from build123d import *

# Parameters (mm, degrees)
SKETCH4_W           = 25
SKETCH4_H           = 25
BOSS_EXTRUDE1_DEPTH = 35
CUT_EXTRUDE12_DEPTH = 50
SKETCH23_W          = 25
SKETCH23_H          = 22.5
CUT_EXTRUDE13_DEPTH = 7
SKETCH24_W          = 30.861916298
SKETCH24_H          = 6.481730837
BOSS_EXTRUDE6_DEPTH = 2
SKETCH25_R          = 1.5
CUT_EXTRUDE14_DEPTH = 3.5
SKETCH26_R          = 1.5
CUT_EXTRUDE15_DEPTH = 3.5
BOSS_EXTRUDE8_DEPTH = 6
SKETCH28_R          = 1.5
CUT_EXTRUDE16_DEPTH = 10
SKETCH29_R          = 1.5
CUT_EXTRUDE17_DEPTH = 10
SKETCH30_R          = 10.5
CUT_EXTRUDE18_DEPTH = 2


with BuildPart() as part:
    # Sketch4 → Boss-Extrude1 (new body)
    with BuildSketch(Plane(origin=(0, 0, 0), x_dir=(1, 0, 0), z_dir=(0, 1, 0))):
        with BuildLine():
            Line((-14.859531773, 13.748687459), (16.140468227, 13.748687459))
            ThreePointArc((16.140468227, 13.748687459), (18.261788571, 12.870007803), (19.140468227, 10.748687459))
            Line((19.140468227, 10.748687459), (19.140468227, -20.251312541))
            ThreePointArc((19.140468227, -20.251312541), (18.261788571, -22.372632884), (16.140468227, -23.251312541))
            Line((16.140468227, -23.251312541), (-14.859531773, -23.251312541))
            ThreePointArc((-14.859531773, -23.251312541), (-16.980852116, -22.372632884), (-17.859531773, -20.251312541))
            Line((-17.859531773, -20.251312541), (-17.859531773, 10.748687459))
            ThreePointArc((-17.859531773, 10.748687459), (-16.980852116, 12.870007803), (-14.859531773, 13.748687459))
        make_face()
        with Locations((0.640468227, -4.751312541)):
            Rectangle(SKETCH4_W, SKETCH4_H, mode=Mode.SUBTRACT)
    extrude(amount=BOSS_EXTRUDE1_DEPTH)

    # Sketch22 → Cut-Extrude12 (cut)
    with BuildSketch(Plane.ZY.offset(17.859531773)):
        Polygon((-13.748687459, 35), (-13.748687459, 0), (13.251312541, 0), (13.251312541, 12), (-1.748687459, 12), (-1.748687459, 6), (-7.748687459, 6), (-7.748687459, 35), align=None)
    extrude(amount=-CUT_EXTRUDE12_DEPTH, mode=Mode.SUBTRACT)

    # Sketch23 → Cut-Extrude13 (cut)
    with BuildSketch(Plane.XY.offset(23.251312541)):
        with Locations((0.640468227, 18.25)):
            Rectangle(SKETCH23_W, SKETCH23_H)
    extrude(amount=-CUT_EXTRUDE13_DEPTH, mode=Mode.SUBTRACT)

    # Sketch24 → Boss-Extrude6 (add)
    with BuildSketch(Plane.XZ):
        with Locations((1.291847829, 16.49217796)):
            Rectangle(SKETCH24_W, SKETCH24_H)
    extrude(amount=-BOSS_EXTRUDE6_DEPTH)

    # Sketch25 → Cut-Extrude14 (cut)
    with BuildSketch(Plane(origin=(0, 0, -7.748687459), x_dir=(-1, 0, 0), z_dir=(0, 0, -1))):
        with Locations((-16.140468227, 21.5)):
            Circle(SKETCH25_R)
        with Locations((-16.140468227, 17)):
            Circle(SKETCH25_R)
        with Locations((-16.140468227, 12.5)):
            Circle(SKETCH25_R)
        with Locations((14.859531773, 12.5)):
            Circle(SKETCH25_R)
        with Locations((14.859531773, 21.5)):
            Circle(SKETCH25_R)
        with Locations((14.859531773, 17)):
            Circle(SKETCH25_R)
        with Locations((14.859531773, 30.5)):
            Circle(SKETCH25_R)
        with Locations((-16.140468227, 30.5)):
            Circle(SKETCH25_R)
        with Locations((-16.140468227, 26)):
            Circle(SKETCH25_R)
        with Locations((14.859531773, 26)):
            Circle(SKETCH25_R)
    extrude(amount=-CUT_EXTRUDE14_DEPTH, mode=Mode.SUBTRACT)

    # Sketch26 → Cut-Extrude15 (cut)
    with BuildSketch(Plane.XZ.offset(-6)):
        with Locations(Location((-14.859531773, -4.748687459, 0), (0, 0, 270))):
            Circle(SKETCH26_R)
        with Locations(Location((16.140468227, -4.748687459, 0), (0, 0, 270))):
            Circle(SKETCH26_R)
    extrude(amount=-CUT_EXTRUDE15_DEPTH, mode=Mode.SUBTRACT)

    # Sketch27 → Boss-Extrude8 (add)
    with BuildSketch(Plane(origin=(0, 35, 0), x_dir=(1, 0, 0), z_dir=(0, 1, 0))):
        with BuildLine():
            Line((-14.859531773, -23.251312541), (16.140468227, -23.251312541))
            ThreePointArc((16.140468227, -23.251312541), (18.261788571, -22.372632884), (19.140468227, -20.251312541))
            Line((19.140468227, -20.251312541), (19.140468227, 10.748687459))
            ThreePointArc((19.140468227, 10.748687459), (18.261788571, 12.870007803), (16.140468227, 13.748687459))
            Line((16.140468227, 13.748687459), (-14.859531773, 13.748687459))
            ThreePointArc((-14.859531773, 13.748687459), (-16.980852116, 12.870007803), (-17.859531773, 10.748687459))
            Line((-17.859531773, 10.748687459), (-17.859531773, -20.251312541))
            ThreePointArc((-17.859531773, -20.251312541), (-16.980852116, -22.372632884), (-14.859531773, -23.251312541))
        make_face()
    extrude(amount=BOSS_EXTRUDE8_DEPTH)

    # Sketch28 → Cut-Extrude16 (cut)
    with BuildSketch(Plane.XY.offset(23.251312541)):
        with Locations((-5.609531773, 32)):
            Circle(SKETCH28_R)
        with Locations((6.890468227, 32)):
            Circle(SKETCH28_R)
        with Locations((-5.609531773, 4.5)):
            Circle(SKETCH28_R)
        with Locations((6.890468227, 4.5)):
            Circle(SKETCH28_R)
    extrude(amount=-CUT_EXTRUDE16_DEPTH, mode=Mode.SUBTRACT)

    # Sketch29 → Cut-Extrude17 (cut)
    with BuildSketch(Plane(origin=(0, 41, 0), x_dir=(1, 0, 0), z_dir=(0, 1, 0))):
        with Locations(Location((0.640468227, 2.248687459, 0), (0, 0, 270))):
            Circle(SKETCH29_R)
        with Locations(Location((7.640468227, -4.751312541, 0), (0, 0, 270))):
            Circle(SKETCH29_R)
        with Locations(Location((0.640468227, -11.751312541, 0), (0, 0, 270))):
            Circle(SKETCH29_R)
        with Locations(Location((-6.359531773, -4.751312541, 0), (0, 0, 270))):
            Circle(SKETCH29_R)
        with Locations(Location((0.640468227, -4.751312541, 0), (0, 0, 270))):
            Circle(SKETCH29_R)
    extrude(amount=-CUT_EXTRUDE17_DEPTH, mode=Mode.SUBTRACT)

    # Sketch30 → Cut-Extrude18 (cut)
    with BuildSketch(Plane(origin=(0, 41, 0), x_dir=(1, 0, 0), z_dir=(0, 1, 0))):
        with Locations(Location((0.640468227, -4.751312541, 0), (0, 0, 270))):
            Circle(SKETCH30_R)
    extrude(amount=-CUT_EXTRUDE18_DEPTH, mode=Mode.SUBTRACT)


solid = part.part
Build history of the part. All positions in model axes, mm. A direction names the side the tool comes from. Round coordinates to 2 decimals unless told otherwise and drop trailing zeros. Loops run counter-clockwise (first coordinate to the right, second up) from the corner with the lowest first, then second, coordinate; pieces in that order, holes last. Notation, with made-up numbers: (66, 32.25) -> (81, 32.25) arc R9 ccw to (81, 40.25) -> close; hole circle Ø6 at (-4.75, 0). An arc over 180 degrees is marked (long way). One line per item, written item: value. Start each with the question number.
Q1. Two-plate mould, pull along Z, no slides. Class faces 4 (the face through (-15, 12, 6)), 5 (the face through (6.176, 37.028, 4.426)), 6 (the face through (16, 17, -4.249)), 7 (the face through (7.58, 30.67, 20.29)): released by +Z, released by -Z, zero draft, split by the parting line, or undercut.
Q2. Cut at D-D on z = 8.5. List the corners of the cut face in (x, y).
Q3. Cut at C-C on x = 7. List the corners of the cut face in (y, z), plus the area to 3 significant figures.
Q4. 3-axis set-ups, long thin cutter, end or side, ignore diameter. For faces 1 (the face through (18.28, 37.96, -12.85)), 2 (the face through (16, 9, -1.749)), 3 (the face through (0, 2, 15)): which of +Z, -Z, +X, -X, +Y, -Y reach the whole face in a straight line?
Q5. Drop flat-ended pins along their axis: pin 1 Ø3.5 at (x, y) = (16, 30.5) entering from -Z; pin 2 Ø3 at (x, z) = (17, 8) entering from -Y; pin 3 Ø1.5 at (x, y) = (-14.5, 25.5) entering from -Z; pin 4 Ø5 at (x, y) = (6.89, 4.5) entering from +Z. Give the stop position or say it passes through.
Q6. Cut at A-A on y = 21.5. List the corners of the cut face in (x, z).
Q7. Cut at B-B on z = 4.5. List the corners of the cut face in (x, y), plus the area to 3 significant figures.
Q8. Probe line 1 along X through (y, z) = (20.5, 4); line 2 along Y through (x, z) = (4, 17); line 3 along Y through (x, z) = (9, 0). List the from-to ranges inside material, lowest first.
Computed:
1. face 4: undercut
1. face 5: undercut
1. face 6: released by -Z
1. face 7: zero draft
2. outline: (-17.86, 12) -> (-11.86, 12) -> (-11.86, 35) -> (13.14, 35) -> (13.14, 12) -> (19.14, 12) -> (19.14, 41) -> (10.45, 41) -> (10.45, 39) -> (-9.17, 39) -> (-9.17, 41) -> (-17.86, 41) -> close
3. outline: (0, 13.25) -> (2, 13.25) -> (2, 17.25) -> (3, 17.25) -> (3, 23.25) -> (0, 23.25) -> close; (6, 17.25) -> (7, 17.25) -> (7, 23.25) -> (6, 23.25) -> close; (29.5, 17.25) -> (30.5, 17.25) -> (30.5, 23.25) -> (29.5, 23.25) -> close; (33.5, 17.25) -> (35, 17.25) -> (35, 6.11) -> (39, 6.11) -> (39, 13.11) -> (41, 13.11) -> (41, 23.25) -> (33.5, 23.25) -> close; (35, -13.75) -> (41, -13.75) -> (41, -3.6) -> (39, -3.6) -> (39, 3.39) -> (35, 3.39) -> close
3. area: 225 mm²
4. face 1: -Z, +X, +Y, -Y
4. face 2: +X, -X, -Y
4. face 3: -Z
5. pin 1: z = -7.75
5. pin 2: y = 12
5. pin 3: z = -4.25
5. pin 4: z = 23.25
6. outline: (-17.86, -7.75) -> (-16.36, -7.75) -> (-16.36, -4.25) -> (-13.36, -4.25) -> (-13.36, -7.75) -> (-11.86, -7.75) -> (-11.86, 23.25) -> (-14.86, 23.25) arc R3 ccw to (-17.86, 20.25) -> close; (13.14, -7.75) -> (14.64, -7.75) -> (14.64, -4.25) -> (17.64, -4.25) -> (17.64, -7.75) -> (19.14, -7.75) -> (19.14, 20.25) arc R3 ccw to (16.14, 23.25) -> (13.14, 23.25) -> close
7. outline: (-17.86, 12) -> (-11.86, 12) -> (-11.86, 35) -> (-7.84, 35) -> (-7.84, 39) -> (-9.86, 39) -> (-9.86, 41) -> (-17.86, 41) -> close; (-4.88, 35) -> (-0.84, 35) -> (-0.84, 39) -> (-4.88, 39) -> close; (2.12, 35) -> (6.16, 35) -> (6.16, 39) -> (2.12, 39) -> close; (9.12, 35) -> (13.14, 35) -> (13.14, 12) -> (19.14, 12) -> (19.14, 41) -> (11.14, 41) -> (11.14, 39) -> (9.12, 39) -> close
7. area: 421 mm²
8. line 1: -17.86 to -11.86, 13.14 to 19.14
8. line 2: 0 to 2, 35 to 41
8. line 3: 35 to 39
